Verification items for the finished model (mm, model axes). Give positions to 0.01 mm unless a question says otherwise; leave off trailing zeros. Order: outer loops, then holes, each group sorted by start corner. A loop starts at its lowest first (then second) coordinate and runs counter-clockwise, first axis right, second up.
from build123d import *

# Parameters (mm, degrees)
SKETCH_1_W          = 20
SKETCH_1_H          = 20
SKETCH_1_W_2        = 18
SKETCH_1_H_2        = 18
EXTRUDE_1_DEPTH     = 438
SKETCH_4_R          = 2
CUT_EXTRUDE_1_DEPTH = 439.912291922


with BuildPart() as part:
    # 草图1 → 拉伸-薄壁1 (new body)
    with BuildSketch(Plane.XY):
        with Locations((10, 10)):
            Rectangle(SKETCH_1_W, SKETCH_1_H)
        with Locations((10, 10)):
            Rectangle(SKETCH_1_W_2, SKETCH_1_H_2, mode=Mode.SUBTRACT)
    extrude(amount=EXTRUDE_1_DEPTH)

    # 草图4 → 切除-拉伸1 (cut, through all)
    with BuildSketch(Plane(origin=(0, 20, 0), x_dir=(1, 0, 0), z_dir=(0, 1, 0))):
        with Locations(Location((5, -413, 0), (0, 0, 270))):
            Circle(SKETCH_4_R)
        with Locations(Location((15, -413, 0), (0, 0, 270))):
            Circle(SKETCH_4_R)
        with Locations(Location((15, -433, 0), (0, 0, 270))):
            Circle(SKETCH_4_R)
        with Locations(Location((5, -433, 0), (0, 0, 270))):
            Circle(SKETCH_4_R)
        with Locations(Location((5, -5, 0), (0, 0, 90))):
            Circle(SKETCH_4_R)
        with Locations(Location((15, -5, 0), (0, 0, 90))):
            Circle(SKETCH_4_R)
        with Locations(Location((15, -25, 0), (0, 0, 90))):
            Circle(SKETCH_4_R)
        with Locations(Location((5, -25, 0), (0, 0, 90))):
            Circle(SKETCH_4_R)
        with Locations(Location((7.5, -149, 0), (0, 0, 270))):
            Circle(SKETCH_4_R)
        with Locations(Location((7.5, -169, 0), (0, 0, 270))):
            Circle(SKETCH_4_R)
        with Locations(Location((7.5, -189, 0), (0, 0, 270))):
            Circle(SKETCH_4_R)
        with Locations(Location((7.5, -209, 0), (0, 0, 270))):
            Circle(SKETCH_4_R)
        with Locations(Location((7.5, -229, 0), (0, 0, 90))):
            Circle(SKETCH_4_R)
        with Locations(Location((7.5, -249, 0), (0, 0, 90))):
            Circle(SKETCH_4_R)
        with Locations(Location((7.5, -269, 0), (0, 0, 90))):
            Circle(SKETCH_4_R)
        with Locations(Location((7.5, -289, 0), (0, 0, 90))):
            Circle(SKETCH_4_R)
    extrude(amount=-CUT_EXTRUDE_1_DEPTH, mode=Mode.SUBTRACT)


solid = part.part
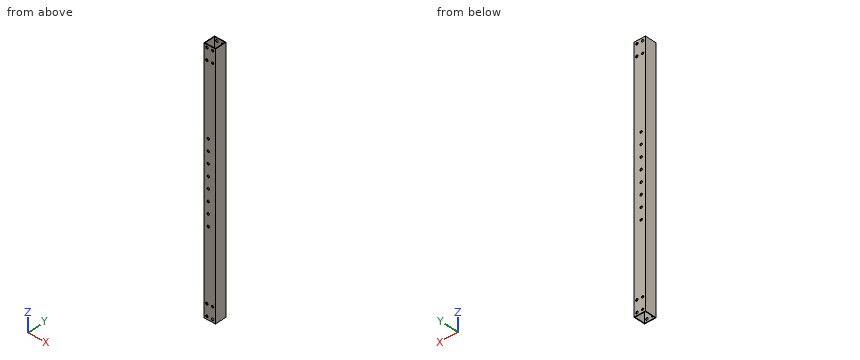
(1) Section check B-B, the plane y = 11.75. Enter the section's corners in (x, z).
Solved:
outline: (0, 0) - (1, 0) - (1, 438) - (0, 438) - close; (19, 0) - (20, 0) - (20, 438) - (19, 438) - close
(2) Scan lines: line 1 (Y direction, x = 13.75, z = 307.5); line 2 (X direction, y = 19.5, z = 5). Record each from-to range of solid material in increasing order.
Solved:
line 1: y = 0 to 1, 19 to 20
line 2: x = 0 to 3, 7 to 13, 17 to 20
(3) Section check A-A, the plane z = 262.5. Enter the section's corners in (x, y).
Solved:
outline: (0, 0) - (20, 0) - (20, 20) - (0, 20) - close; hole (1, 1) - (19, 1) - (19, 19) - (1, 19) - close
